Input: dimensioned drawing with shaded views. Units: mm. Origin: part minimum x, y, z. A direction names the side the tool comes from. Coordinates: 2 decimals unless noted, no trailing zeros. Order: outer loops, then holes, each group sorted by start corner. A loop starts at its lowest first (then second) coordinate and runs counter-clockwise, first axis right, second up. Notation, with made-up numbers: (-27.75, -11.75) -> (-11.75, -11.75) arc R14 ccw to (-11.75, 8.25) -> close; hole circle Ø9 at (45.5, -3). An arc over 180 degrees is marked (long way). Answer as CSV lines item,"result".
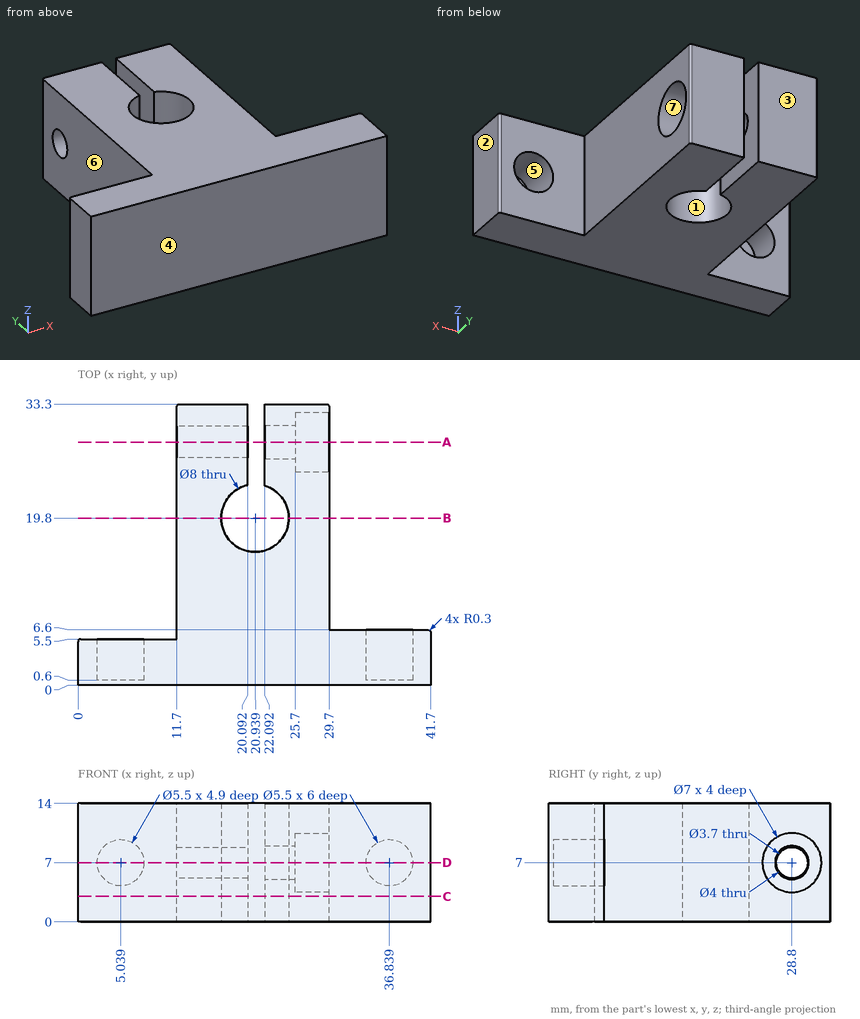
1. Cut plane D-D (z = 7). State how many separate pieces and enclosed holes the cut face has, plus the area to 3 significant figures.
Findings:
separate pieces,"3"
enclosed holes,"0"
area,"540 mm2"
2. Cut plane C-C (z = 3). Return the cut outline in (x, y).
Findings:
outline,"(0, 0) -> (41.7, 0) -> (41.7, 6.3) arc R0.3 ccw to (41.4, 6.6) -> (29.7, 6.6) -> (29.7, 33) arc R0.3 ccw to (29.4, 33.3) -> (22.09, 33.3) -> (22.09, 23.63) arc R4 cw (long way) to (20.09, 23.71) -> (20.09, 33.3) -> (12, 33.3) arc R0.3 ccw to (11.7, 33) -> (11.7, 5.5) -> (0.3, 5.5) arc R0.3 ccw to (0, 5.2) -> close"
3. Ray query, line 1 along X through (y, z) = (27, 8.75); line 2 along X through (y, z) = (19.8, 3.5); line 3 along X through (y, z) = (3.6, 7). Return the intervals inside material, ascending.
Findings:
line 1,"x = 11.7 to 20.09, 22.09 to 25.7"
line 2,"x = 11.7 to 16.94, 24.94 to 29.7"
line 3,"x = 0 to 2.29, 7.79 to 34.09, 39.59 to 41.7"
4. Cut plane A-A (y = 28.8). Return the cut outline in (x, z).
Findings:
outline,"(11.7, 0) -> (20.09, 0) -> (20.09, 5.15) -> (11.7, 5.15) -> close; (11.7, 8.85) -> (20.09, 8.85) -> (20.09, 14) -> (11.7, 14) -> close; (22.09, 0) -> (29.7, 0) -> (29.7, 3.5) -> (25.7, 3.5) -> (25.7, 5) -> (22.09, 5) -> close; (22.09, 9) -> (25.7, 9) -> (25.7, 10.5) -> (29.7, 10.5) -> (29.7, 14) -> (22.09, 14) -> close"
5. Mould query, pull axis Y, two halves, no side actions, for the marked faces 1, 2, 3 and 4. Classes: released by +Y, released by -Y, zero draft, split by the parting line, or undercut.
Findings:
face 1,"undercut"
face 2,"zero draft"
face 3,"released by +Y"
face 4,"released by -Y"
6. Cut plane B-B (y = 19.8). Return the cut outline in (x, z), plus the area to 3 significant figures.
Findings:
outline,"(11.7, 0) -> (16.94, 0) -> (16.94, 14) -> (11.7, 14) -> close; (24.94, 0) -> (29.7, 0) -> (29.7, 14) -> (24.94, 14) -> close"
area,"140 mm2"
7. Contact query for flat-ended pins moving along their axis: pin 1 (3 mm diameter, centred on y = 26.5, z = 8, fed in from -X); pin 2 (2 mm diameter, centred on y = 30.5, z = 6.5, fed in from +X); pin 3 (6 mm diameter, centred on x = 6, z = 6, fed in from +Y); pin 4 (3 mm diameter, centred on y = 28.8, z = 7, fed in from -X). Output: stop coordinate, or through.
Findings:
pin 1,"stops at x = 11.7"
pin 2,"stops at x = 25.7"
pin 3,"stops at y = 5.5"
pin 4,"passes through"
8. Reachability of the marked faces 5, 6 and 7 from +Z, -Z, +X, -X, +Y, -Y: full face, straight path, thin tool, end or side. Return the list, or none.
Findings:
face 5,"+Y"
face 6,"+Z, -Z, -X, +Y"
face 7,"+X"
